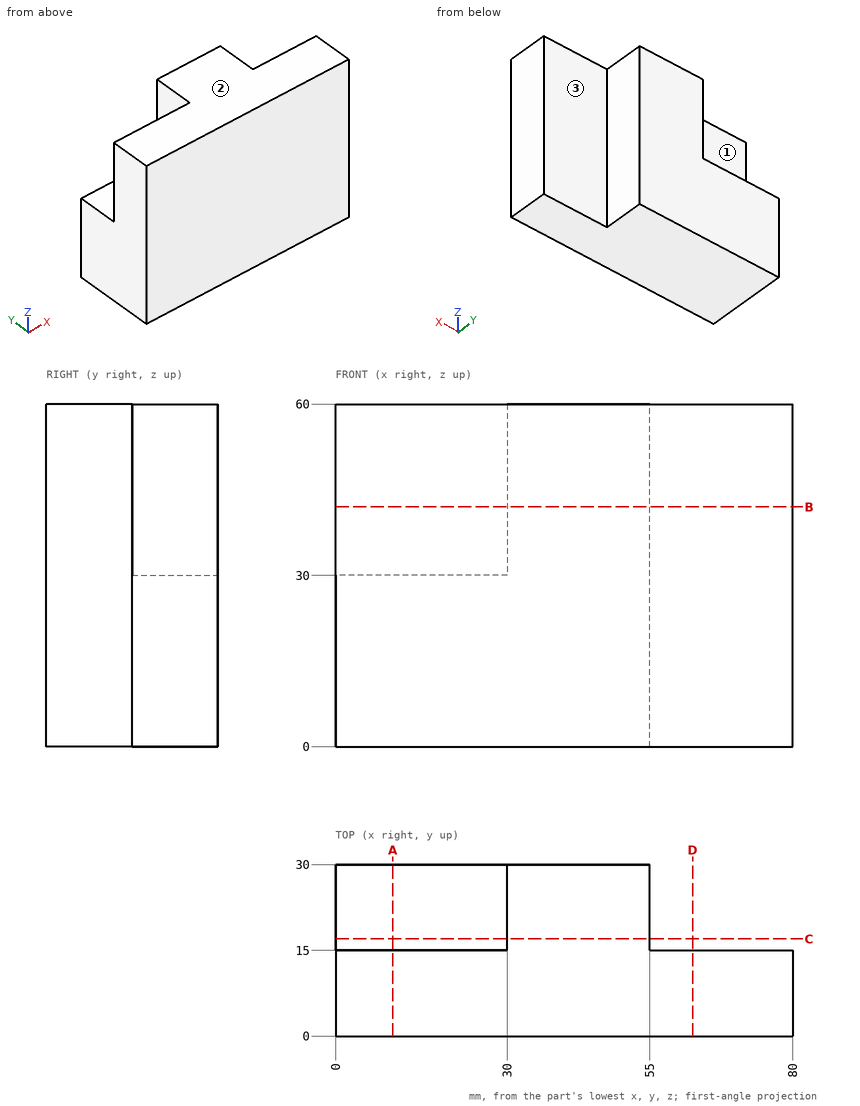
Check sheet for the drawn part. Datum: minimum x, y, z corner. Units: mm. A direction names the side the tool comes from. Round coordinates to 2 decimals unless told otherwise and drop trailing zeros. Write each loop counter-clockwise with the first axis right and the second up, starting at its lowest first coordinate (ties: lowest second). Pieces come first, ordered by that corner, then holes. Notation, with made-up numbers: (3, 47.5) -> (42, 47.5) arc R23 cw to (42, 85.5) -> close; hole circle Ø5 at (24, 67.5). An arc over 180 degrees is marked (long way). Write each question's results on one line, items separated by ' | '. Start each with the question number.
1. Depth check by flat-ended pin: P1, Ø7.5, axis at y = 21, z = 21.5, coming from the +X side; P2, Ø7.5, axis at x = 11, y = 20, coming from the +Z side; P3, Ø3, axis at y = 27, z = 51, coming from the -X side. Enter the tip coordinate at first touch or a pass-through.
2. Cross-section at A-A (x = 10). Enter the section's corners in (y, z).
3. Cross-section at D-D (x = 62.5). Enter the section's corners in (y, z).
4. Cross-section at C-C (y = 17). Enter the section's corners in (x, z).
5. Cross-section at B-B (z = 42). Enter the section's corners in (x, y), then the cut area to 4 significant figures.
6. Set-up check for the marked faces 1, 2 and 3: record each of +Z, -Z, +X, -X, +Y, -Y from which the full face is reachable in a straight line by a thin tool's end or side.
7. Material ranges on probe 1 along Y at (x, z) = (16, 42); probe 2 along Z at (x, y) = (23, 16.5); probe 3 along X at (y, z) = (19.25, 57.5), recorded low to high. Write a range as from..to.
Solutions:
1) P1: stops at x = 55 | P2: stops at z = 30 | P3: stops at x = 30
2) outline: (0, 0) -> (30, 0) -> (30, 30) -> (15, 30) -> (15, 60) -> (0, 60) -> close
3) outline: (0, 0) -> (15, 0) -> (15, 60) -> (0, 60) -> close
4) outline: (0, 0) -> (55, 0) -> (55, 60) -> (30, 60) -> (30, 30) -> (0, 30) -> close
5) outline: (0, 0) -> (80, 0) -> (80, 15) -> (55, 15) -> (55, 30) -> (30, 30) -> (30, 15) -> (0, 15) -> close | area: 1,575 mm2
6) face 1: +Z, -X, +Y | face 2: +Z, +X, -X, +Y, -Y | face 3: +Z, -Z, +X, +Y
7) probe 1: y = 0..15 | probe 2: z = 0..30 | probe 3: x = 30..55
